Check sheet for the modelled part. Datum: model origin and axes. Units: mm. Face numbers are marked on the shaded views. Coordinates: 2 decimals unless noted, no trailing zeros. Order: outer loops, then holes, each group sorted by start corner. A loop starts at its lowest first (then second) coordinate and runs counter-clockwise, first axis right, second up.
Autodesk Inventor part; units mm, degrees
ref_plane "YZ Plane" through (0, 0, 0) normal (1, 0, 0) x (0, 1, 0)
ref_plane "XZ Plane" through (0, 0, 0) normal (0, 1, 0) x (-1, 0, 0)
ref_plane "XY Plane" through (0, 0, 0) normal (0, 0, 1) x (1, 0, 0)
sketch "Sketch1" plane through (0, 0, 0) normal (0, 0, 1) x (1, 0, 0)
  line L0 (-9.677, -30.5907) -> (-13.477, -30.5907)
  line L1 (-9.677, -30.5907) -> (-9.677, -46.5907)
  line L2 (-9.677, -46.5907) -> (-11.677, -46.5907)
  line L3 (-11.677, -46.5907) -> (-11.677, -30.5907)
  line L4 (-9.677, -30.5907) -> (-9.677, -26.5988)
  line L5 (-13.477, -30.5907) -> (-13.477, -30.2107)
  line L6 (-13.477, -30.2107) -> (-13.477, -28.3907)
  line L7 (-13.477, -28.3907) -> (-9.677, -28.3907)
  point P0 (0, 0)
  dimension "d0" = 3.8
  dimension "d2" = 16
  dimension "d3" = 2
  dimension "d18" = 0.38
  dimension "d19" = 2.2
revolve "Revolution1" add sketch "Sketch1" angle 360 about axis through (-9.677, -30.5907, 0) along (0, -1, 0)
chamfer "Chamfer2" distance 0.2 angle 45 1 edges at (-7.677, -46.5907, 0)
thread "Rosca1"
fillet "Empalme2" radius 1.82 1 edges at (-5.877, -28.3907, 0)
sketch "Boceto2" plane through (-9.677, -28.3907, 0) normal (0, 1, 0) x (1, 0, 0)
  line L0 (1.1232, 0.9065) -> (1.3467, -0.5194)
  line L1 (1.3467, -0.5194) -> (0.2235, -1.426)
  line L2 (0.2235, -1.426) -> (-1.1232, -0.9065)
  line L3 (-1.1232, -0.9065) -> (-1.3467, 0.5194)
  line L4 (-1.3467, 0.5194) -> (-0.2235, 1.426)
  line L5 (-0.2235, 1.426) -> (1.1232, 0.9065)
  point P0 (9.677, 0)
  point P1 (0, 0)
  dimension "d21" = 2.5
extrude "Extrusión1" cut sketch "Boceto2" against normal blind 1.3
properties part number "Tornillo Allen cabeza botón M4x16mm"
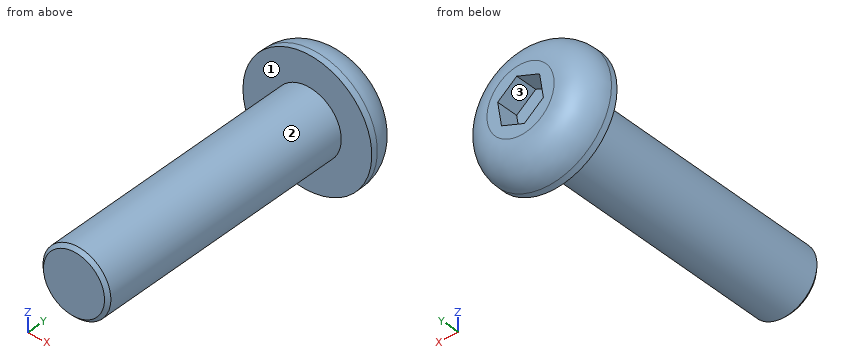
(1) Go/stop test with a flat-tipped pin: P1, Ø0.8, axis at x = -10, z = 0.5, coming from the +Y side. Record where the tip stops, or that it passes through.
Filled in:
P1: stops at y = -29.69
(2) Thickness scan on probe 1 along Z at (x, y) = (-9.75, -39.25); probe 2 along Y at (x, z) = (-10.25, -2); probe 3 along Y at (x, z) = (-10, 0.25). Record the ranges inside material, lowest first.
Filled in:
probe 1: z = -2 to 2
probe 2: y = -30.59 to -28.39
probe 3: y = -46.59 to -29.69
(3) Release check for a two-part mould opening along Z. For the marked faces 1, 2 and 3 record: +Z half, -Z half, draft (parallel to the pull), parting line (faces both ways), or undercut.
Filled in:
face 1: draft
face 2: parting line
face 3: undercut
(4) Cross-section at A-A (y = -33.25). Enter the section's corners in (x, z).
Filled in:
outline: circle Ø4 at (-9.68, 0)
